```python
from build123d import *

# Parameters (mm, degrees)
F1_DEPTH = 5
F3_D     = 2.5
F3_DEPTH = 3
F3_TIP   = 0.7510757738
F4_R     = 1.375
F5_DEPTH = 6
F6_SIZE  = 0.25


with BuildPart() as f1:
    # F0 (on Top) → F1 (new body)
    with BuildSketch(Plane.XY):
        Polygon((1.3423393759, 2.325), (-1.3423393759, 2.325), (-2.6846787517, 0), (-1.3423393759, -2.325), (1.3423393759, -2.325), (2.6846787517, 0), align=None)
    extrude(amount=F1_DEPTH)

    # F3
    with Locations(Plane.XY.offset(5)):
        with Locations((0, 0)):
            Hole(F3_D / 2, depth=F3_DEPTH)
            with Locations((0, 0, -(F3_DEPTH + F3_TIP / 2))):  # 118° drill point
                Cone(0, F3_D / 2, F3_TIP, mode=Mode.SUBTRACT)

    # F4 (on face) → F5 (join)
    with BuildSketch(Plane(origin=(0, 0, 0), x_dir=(1, 0, 0), z_dir=(0, 0, -1))):
        Circle(F4_R)
    extrude(amount=F5_DEPTH)

    # F6
    f6_edges = [f1.edges().sort_by_distance(p)[0] for p in [
        (-1.375, 0, -6),
    ]]
    chamfer(f6_edges, length=F6_SIZE)


solid = f1.part
```
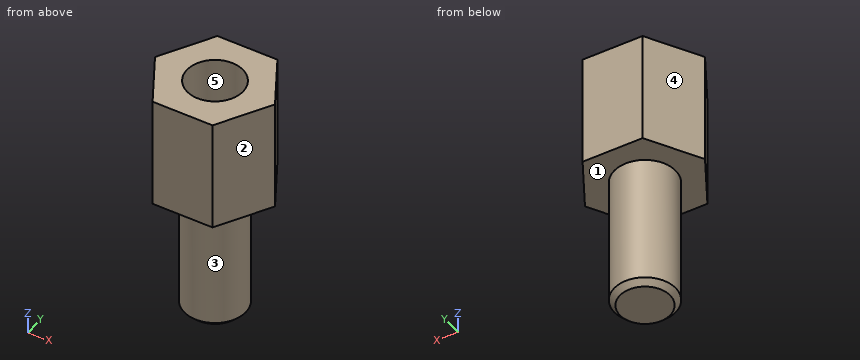
Model file for the job. Use its own axes, mm. Face numbers are marked on the shaded views. A direction names the side the tool comes from. Coordinates: 2 decimals unless noted, no trailing zeros. Write each loop counter-clockwise with the first axis right and the second up, starting at its lowest first coordinate (ties: lowest second). Pieces come first, ordered by that corner, then holes. Notation, with made-up numbers: (15, 47) - (56, 47) arc R22 ccw to (56, 79) - close; hole circle Ø1 at (39, 16). An arc over 180 degrees is marked (long way). One line per question, with ' | ' between items. Start each with the question number.
Q1. Cut at D-D, the plane z = 1.5. List the corners of the cut face in (x, y) (3 decimals), then the cut area to 3 significant figures.
Q2. Cut at C-C, the plane z = -2.75. List the corners of the cut face in (x, y) (3 decimals).
Q3. Cut at A-A, the plane z = 4. List the corners of the cut face in (x, y) (3 decimals), then the cut area to 3 significant figures.
Q4. Pull direction X, two halves, no side cores. Call the marked faces 3, 4 and 5: pulls with the +X half, pulls with the -X half, needs draft (parallel to the pull), parting line crosses it, or undercut.
Q5. Cut at B-B, the plane y = -1.55. List the corners of the cut face in (x, z), then the cut area to 3 significant figures.
Q6. Drill centre lines: line 1 (Y direction, x = 0, z = 4.3) (3 decimals); line 2 (Z direction, x = -0.25, y = -1.9); line 3 (X direction, y = -0.35, z = 3.25). Where is each one in solid material? Low to high. Write a range as [from, to].
Q7. 3-axis set-ups, long thin cutter, end or side, ignore diameter. For the marked faces 1 and 2: which of +Z, -Z, +X, -X, +Y, -Y reach the whole face in a straight line?
Answer below:
1) outline: (-2.685, 0) - (-1.342, -2.325) - (1.342, -2.325) - (2.685, 0) - (1.342, 2.325) - (-1.342, 2.325) - close; hole circle Ø0.836 at (0, 0) | area: 18.2 mm^2
2) outline: circle Ø2.75 at (0, 0)
3) outline: (-2.685, 0) - (-1.342, -2.325) - (1.342, -2.325) - (2.685, 0) - (1.342, 2.325) - (-1.342, 2.325) - close; hole circle Ø2.5 at (0, 0) | area: 13.8 mm^2
4) face 3: parting line crosses it | face 4: pulls with the -X half | face 5: undercut
5) outline: (-1.79, 0) - (1.79, 0) - (1.79, 5) - (-1.79, 5) - close | area: 17.9 mm^2
6) line 1: [-2.325, -1.25], [1.25, 2.325] | line 2: [0, 5] | line 3: [-2.48, -1.2], [1.2, 2.48]
7) face 1: -Z | face 2: +Z, -Z, +X, -Y
